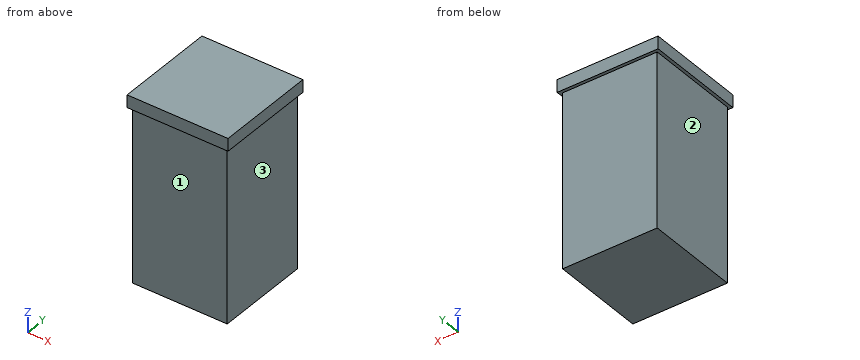
from build123d import *

# Parameters (mm, degrees)
SKETCH1_W           = 48
SKETCH1_H           = 48
BOSS_EXTRUDE1_DEPTH = 6
SKETCH2_W           = 45
SKETCH2_H           = 45
BOSS_EXTRUDE2_DEPTH = 82.75


with BuildPart() as part:
    # Sketch1 → Boss-Extrude1 (new body)
    with BuildSketch(Plane.XY):
        Rectangle(SKETCH1_W, SKETCH1_H)
    extrude(amount=-BOSS_EXTRUDE1_DEPTH)

    # Sketch2 → Boss-Extrude2 (add)
    with BuildSketch(Plane(origin=(0, 0, -6), x_dir=(-1, 0, 0), z_dir=(0, 0, -1))):
        Rectangle(SKETCH2_W, SKETCH2_H)
    extrude(amount=BOSS_EXTRUDE2_DEPTH)


solid = part.part
Can you work these out from the model? Positions are in its coordinate system, mm. Face numbers are marked on the shaded views. A direction names the side the tool comes from. Coordinates: 2 decimals unless noted, no trailing zeros. Write each loop counter-clockwise with the first axis right and the second up, starting at its lowest first coordinate (ties: lowest second). Pieces come first, ordered by that corner, then holes. Notation, with made-up numbers: (-18, 43.25) -> (39, 43.25) arc R4 ccw to (39, 49.25) -> close; hole circle Ø8 at (-7, 86). An arc over 180 degrees is marked (long way). Write each question's results on one line, items separated by ' | '. Start each with the question number.
Q1. On a 3-axis mill with a long thin cutter (end or side, diameter ignored), from which of +Z, -Z, +X, -X, +Y, -Y can I reach the whole of each face in a straight line? I mean the marked faces 1, 2 and 3. Say none if no direction works.
Q2. Imagine slicing it at C-C (z = -76). Write out the boundary of the cut face in (x, y), then the cut area to 4 significant figures.
Q3. If I drill on probe 1 along X at (y, z) = (11, -31.5), over which ranges is the centre line in solid material (lowest first)?
Q4. Imagine slicing it at A-A (x = 10). Write out the boundary of the cut face in (y, z).
Q5. I'm going to push flat-ended pins straight in: pin 1 (4 mm diameter, centred on y = 18.5, z = -35, fed in from +X); pin 2 (5 mm diameter, centred on x = 4, z = -16.5, fed in from +Y); pin 3 (1 mm diameter, centred on x = 14, z = -20.5, fed in from -Y). Where does each tip first touch, or does it pass through?
Taken from the geometry:
1) face 1: -Z, +X, -X, -Y | face 2: -Z, -X, +Y, -Y | face 3: -Z, +X, +Y, -Y
2) outline: (-22.5, -22.5) -> (22.5, -22.5) -> (22.5, 22.5) -> (-22.5, 22.5) -> close | area: 2,025 mm^2
3) probe 1: x = -22.5 to 22.5
4) outline: (-24, -6) -> (-22.5, -6) -> (-22.5, -88.75) -> (22.5, -88.75) -> (22.5, -6) -> (24, -6) -> (24, 0) -> (-24, 0) -> close
5) pin 1: stops at x = 22.5 | pin 2: stops at y = 22.5 | pin 3: stops at y = -22.5
